Model file for the job. Use its own axes, mm. A direction names the side the tool comes from. Give positions to 0.01 mm unless a question says otherwise; leave off trailing zeros. Order: outer loops, then holes, each group sorted by start corner. A loop starts at its lowest first (then second) coordinate and runs counter-clockwise, first axis right, second up. Notation, with made-up numbers: M 3.5,-20 L 36.5,-20 A16 cw 36.5,-6 Z; hole C 46.25,80 d6. An arc over 180 degrees is marked long. Return JSON: item names as keys, results as strings. Group by question number.
1. Wall check: probe 1 along Z at (x, y) = (5.75, 2); probe 2 along X at (y, z) = (-4.4, 14.5); probe 3 along Z at (x, y) = (-10, 2.5). Give the ranges that are in metal, low to high. Write a range as [from, to].
2. Two-plate mould, pull along Y, no slides. Class faces 5 (the face through (7.5, -2.02, 15.97)), 6 (the face through (0, -6.5, 14)), 7 (the face through (0, 0, 2)), 8 (the face through (11, -0.5, 16)): released by +Y, released by -Y, zero draft, split by the parting line, or undercut.
3. Slice it at A-A on z = 12.5. List the corners of the cut face in (x, y), then the cut area to 3 significant figures.
4. 3-axis set-ups, long thin cutter, end or side, ignore diameter. For faces 1 (the face through (-1, -3, 7)), 2 (the face through (-10.97, -5.02, 13.23)), 3 (the face through (-7.477, -2.021, 15.93)), 4 (the face through (11, -2, 17.4)): which of +Z, -Z, +X, -X, +Y, -Y reach the whole face in a straight line?
5. Pin check, flat tips, straight feed: pin 1 (3 mm diameter, centred on x = 1.5, z = 12.5, fed in from +Y); pin 2 (0.9 mm diameter, centred on x = 12, y = -1.5, fed in from -Z); pin 3 (2.5 mm diameter, centred on x = -9.5, y = -2, fed in from +Z). Stop position of each tip, or through.
6. Slice it at B-B on z = 24.5. Give the number of separate pieces and of enclosed holes in the cut face, then the cut area to 3 significant figures.
from build123d import *

# Parameters (mm, degrees)
ESBO_O1_W                  = 26
ESBO_O1_H                  = 13
RESSALTO_EXTRUS_O1_DEPTH   = 29
CORTE_EXTRUS_O1_DEPTH      = 33.438403167
CORTE_EXTRUS_O1_DEPTH_BACK = 33.438403167
ESBO_O2_R                  = 5.5
ESBO_O3_R                  = 7.5
CORTE_EXTRUS_O2_DEPTH      = 25
CORTE_EXTRUS_O3_DEPTH      = 35.336569427
CORTE_EXTRUS_O3_DEPTH_BACK = 35.336569427
ESBO_O4_R                  = 1.6
CORTE_EXTRUS_O4_DEPTH      = 3
ESBO_O9_W                  = 8
ESBO_O9_H                  = 4
CORTE_EXTRUS_O5_DEPTH      = 3
FILETE1_R                  = 5


with BuildPart() as part:
    # Esboço1 → Ressalto-extrusão1 (new body)
    with BuildSketch(Plane.XY):
        Rectangle(ESBO_O1_W, ESBO_O1_H)
    extrude(amount=RESSALTO_EXTRUS_O1_DEPTH)

    # Esboço2 → Corte-extrusão1 (cut, two sides: drawn at the far end of the back side and taken through both)
    with BuildSketch(Plane.XY.offset(29).offset(-CORTE_EXTRUS_O1_DEPTH_BACK)):
        with Locations((0, 6.5)):
            Circle(ESBO_O2_R)
    extrude(amount=CORTE_EXTRUS_O1_DEPTH + CORTE_EXTRUS_O1_DEPTH_BACK, mode=Mode.SUBTRACT)

    # Esboço3 → Corte-extrusão2 (cut)
    with BuildSketch(Plane.XY.offset(27)):
        with Locations((0, 6.5)):
            Circle(ESBO_O3_R)
    extrude(amount=-CORTE_EXTRUS_O2_DEPTH, mode=Mode.SUBTRACT)

    # Esboço4 → Corte-extrusão3 (cut, two sides: drawn at the far end of the back side and taken through both)
    with BuildSketch(Plane(origin=(0, 6.5, 0), x_dir=(1, 0, 0), z_dir=(0, 1, 0)).offset(-CORTE_EXTRUS_O3_DEPTH_BACK)):
        with Locations(Location((-10, -14.5, 0), (0, 0, 270))):
            Circle(ESBO_O4_R)
        with Locations(Location((10, -14.5, 0), (0, 0, 270))):
            Circle(ESBO_O4_R)
    extrude(amount=CORTE_EXTRUS_O3_DEPTH + CORTE_EXTRUS_O3_DEPTH_BACK, mode=Mode.SUBTRACT)

    # Varredura de corte3: read off the stored shape, not the designer's step
    # Varredura de corte3: loft between two sections, ruled curve by curve
    varredura_de_corte3_from = [
        Edge.make_bspline([(-10.775531387, 11.14102753, 3), (-10.815047893, 10.387007675, 3), (-10.859579119, 9.537232339, 3), (-10.942482774, 7.955474229, 3), (-11.000003483, 7.230191203, 3), (-10.999993175, 5.06927711, 3), (-10.717078713, 3.385508213, 3), (-9.067866438, -0.006108266, 3), (-7.679635371, -1.685716419, 3), (-4.830903728, -3.44525385, 3), (-3.774716833, -3.895333549, 3), (-1.552511027, -4.449938605, 3), (-0.403453822, -4.550209028, 3), (2.969944564, -4.328615808, 3), (5.023571546, -3.476580102, 3), (8.13506471, -1.154366891, 3), (9.189674801, 0.267167465, 3), (10.533085234, 2.985384839, 3), (10.837160801, 4.285623822, 3), (11.004780041, 6.01871971, 3), (11.006990461, 6.575860832, 3), (10.96949773, 7.517101654, 3), (10.943022714, 7.945129378, 3), (10.873144208, 9.27841043, 3), (10.824758408, 10.201720017, 3), (10.775531387, 11.14102753, 3)], [0, 0, 0, 0, 0.056576928, 0.056576928, 0.113153857, 0.113153857, 0.224009625, 0.224009625, 0.334865393, 0.334865393, 0.390293276, 0.390293276, 0.44572116, 0.44572116, 0.556576928, 0.556576928, 0.667432696, 0.667432696, 0.778288464, 0.778288464, 0.833716348, 0.833716348, 0.889144232, 0.889144232, 1, 1, 1, 1], 3),
        Edge.make_bspline([(-8.778272317, 11.036355618, 3), (-8.818366558, 10.271311923, 3), (-8.86155068, 9.447238277, 3), (-8.945993073, 7.836124466, 3), (-9.000002401, 7.107268908, 3), (-8.999995296, 5.310128738, 3), (-8.764237068, 3.942975251, 3), (-7.423445328, 1.185624705, 3), (-6.27357029, -0.203437636, 3), (-3.957441466, -1.63400923, 3), (-3.084493861, -2.006248941, 3), (-1.274147115, -2.45806464, 3), (-0.32387933, -2.540671478, 3), (2.417516141, -2.360593842, 3), (4.119219834, -1.655921663, 3), (6.646937102, 0.230601396, 3), (7.51801706, 1.398774697, 3), (8.618786605, 3.626040825, 3), (8.867342653, 4.694186327, 3), (9.003623581, 6.103250891, 3), (9.006690622, 6.5435831, 3), (8.972969022, 7.390126226, 3), (8.946060492, 7.834793966, 3), (8.875291444, 9.185065517, 3), (8.82794518, 10.088540932, 3), (8.778272317, 11.036355618, 3)], [0, 0, 0, 0, 0.056576928, 0.056576928, 0.113153857, 0.113153857, 0.224009625, 0.224009625, 0.334865393, 0.334865393, 0.390293276, 0.390293276, 0.44572116, 0.44572116, 0.556576928, 0.556576928, 0.667432696, 0.667432696, 0.778288464, 0.778288464, 0.833716348, 0.833716348, 0.889144232, 0.889144232, 1, 1, 1, 1], 3),
        Edge.make_line((-8.778272317, 11.036355618, 3), (-10.775531387, 11.14102753, 3)),
        Edge.make_line((8.778272317, 11.036355618, 3), (10.775531387, 11.14102753, 3)),
    ]
    varredura_de_corte3_to = [
        Edge.make_bspline([(-10.775531387, 11.14102753, 7), (-10.815047893, 10.387007675, 7), (-10.859579119, 9.537232339, 7), (-10.942482774, 7.955474229, 7), (-11.000003483, 7.230191203, 7), (-10.999993175, 5.06927711, 7), (-10.717078713, 3.385508213, 7), (-9.067866438, -0.006108266, 7), (-7.679635371, -1.685716419, 7), (-4.830903728, -3.44525385, 7), (-3.774716833, -3.895333549, 7), (-1.552511027, -4.449938605, 7), (-0.403453822, -4.550209028, 7), (2.969944564, -4.328615808, 7), (5.023571546, -3.476580102, 7), (8.13506471, -1.154366891, 7), (9.189674801, 0.267167465, 7), (10.533085234, 2.985384839, 7), (10.837160801, 4.285623822, 7), (11.004780041, 6.01871971, 7), (11.006990461, 6.575860832, 7), (10.96949773, 7.517101654, 7), (10.943022714, 7.945129378, 7), (10.873144208, 9.27841043, 7), (10.824758408, 10.201720017, 7), (10.775531387, 11.14102753, 7)], [0, 0, 0, 0, 0.056576928, 0.056576928, 0.113153857, 0.113153857, 0.224009625, 0.224009625, 0.334865393, 0.334865393, 0.390293276, 0.390293276, 0.44572116, 0.44572116, 0.556576928, 0.556576928, 0.667432696, 0.667432696, 0.778288464, 0.778288464, 0.833716348, 0.833716348, 0.889144232, 0.889144232, 1, 1, 1, 1], 3),
        Edge.make_bspline([(-8.778272317, 11.036355618, 7), (-8.818366558, 10.271311923, 7), (-8.86155068, 9.447238277, 7), (-8.945993073, 7.836124466, 7), (-9.000002401, 7.107268908, 7), (-8.999995296, 5.310128738, 7), (-8.764237068, 3.942975251, 7), (-7.423445328, 1.185624705, 7), (-6.27357029, -0.203437636, 7), (-3.957441466, -1.63400923, 7), (-3.084493861, -2.006248941, 7), (-1.274147115, -2.45806464, 7), (-0.32387933, -2.540671478, 7), (2.417516141, -2.360593842, 7), (4.119219834, -1.655921663, 7), (6.646937102, 0.230601396, 7), (7.51801706, 1.398774697, 7), (8.618786605, 3.626040825, 7), (8.867342653, 4.694186327, 7), (9.003623581, 6.103250891, 7), (9.006690622, 6.5435831, 7), (8.972969022, 7.390126226, 7), (8.946060492, 7.834793966, 7), (8.875291444, 9.185065517, 7), (8.82794518, 10.088540932, 7), (8.778272317, 11.036355618, 7)], [0, 0, 0, 0, 0.056576928, 0.056576928, 0.113153857, 0.113153857, 0.224009625, 0.224009625, 0.334865393, 0.334865393, 0.390293276, 0.390293276, 0.44572116, 0.44572116, 0.556576928, 0.556576928, 0.667432696, 0.667432696, 0.778288464, 0.778288464, 0.833716348, 0.833716348, 0.889144232, 0.889144232, 1, 1, 1, 1], 3),
        Edge.make_line((-8.778272317, 11.036355618, 7), (-10.775531387, 11.14102753, 7)),
        Edge.make_line((8.778272317, 11.036355618, 7), (10.775531387, 11.14102753, 7)),
    ]
    varredura_de_corte3 = Solid(Shell([*[Face.make_surface_from_curves(varredura_de_corte3_from[k], varredura_de_corte3_to[k]) for k in range(4)], Face(Wire(varredura_de_corte3_from)), Face(Wire(varredura_de_corte3_to))]))
    add(varredura_de_corte3, mode=Mode.SUBTRACT)

    # Varredura de corte3 2: loft between two sections, ruled curve by curve
    varredura_de_corte3_2_from = [
        Edge.make_bspline([(-10.775531387, 11.14102753, 22), (-10.815050253, 10.386962648, 22), (-10.859635544, 9.536156226, 22), (-10.942604964, 7.953142141, 22), (-11.000003387, 7.227604876, 22), (-10.999993448, 5.09243912, 22), (-10.726075216, 3.44374676, 22), (-9.146415207, 0.117814577, 22), (-7.826638231, -1.531050563, 22), (-4.171497206, -3.909251659, 22), (-1.912358031, -4.556779213, 22), (2.517456834, -4.434897746, 22), (4.570919991, -3.689422793, 22), (7.764052722, -1.527285148, 22), (8.887440792, -0.158899703, 22), (10.364225069, 2.511206921, 22), (10.732123337, 3.816518914, 22), (10.975605623, 5.5614094, 22), (11.004902153, 6.119453759, 22), (10.993656399, 7.13678057, 22), (10.963259766, 7.559009248, 22), (10.895302463, 8.855554069, 22), (10.847393897, 9.769809145, 22), (10.799382035, 10.685930053, 22)], [0, 0, 0, 0, 0.057220999, 0.057220999, 0.114441998, 0.114441998, 0.225136749, 0.225136749, 0.335831499, 0.335831499, 0.446526249, 0.446526249, 0.557220999, 0.557220999, 0.667915749, 0.667915749, 0.7786105, 0.7786105, 0.833957875, 0.833957875, 0.88930525, 0.88930525, 1, 1, 1, 1], 3),
        Edge.make_bspline([(-8.778272317, 11.036355618, 22), (-8.818364203, 10.271356871, 22), (-8.861613386, 9.446042366, 22), (-8.946108983, 7.833912176, 22), (-9.000002332, 7.104831646, 22), (-8.999995488, 5.329945493, 22), (-8.772011309, 3.991285732, 22), (-7.487299037, 1.286355363, 22), (-6.385007619, -0.082964565, 22), (-3.431648648, -2.004555434, 22), (-1.541287594, -2.5458131, 22), (2.036368433, -2.447377138, 22), (3.749427608, -1.830311698, 22), (6.342822793, -0.074267526, 22), (7.271131746, 1.051066146, 22), (8.480231231, 3.237185214, 22), (8.780527991, 4.302274211, 22), (8.980191062, 5.733137414, 22), (9.004131059, 6.178194136, 22), (8.994672137, 7.033801275, 22), (8.966591972, 7.443057915, 22), (8.896860843, 8.773440999, 22), (8.851022767, 9.64819435, 22), (8.802122965, 10.58125814, 22)], [0, 0, 0, 0, 0.057220999, 0.057220999, 0.114441998, 0.114441998, 0.225136749, 0.225136749, 0.335831499, 0.335831499, 0.446526249, 0.446526249, 0.557220999, 0.557220999, 0.667915749, 0.667915749, 0.7786105, 0.7786105, 0.833957875, 0.833957875, 0.88930525, 0.88930525, 1, 1, 1, 1], 3),
        Edge.make_line((-8.778272317, 11.036355618, 22), (-10.775531387, 11.14102753, 22)),
        Edge.make_line((8.802122965, 10.58125814, 22), (10.799382035, 10.685930053, 22)),
    ]
    varredura_de_corte3_2_to = [
        Edge.make_bspline([(-10.775531387, 11.14102753, 26), (-10.815050253, 10.386962648, 26), (-10.859635544, 9.536156226, 26), (-10.942604964, 7.953142141, 26), (-11.000003387, 7.227604876, 26), (-10.999993448, 5.09243912, 26), (-10.726075216, 3.44374676, 26), (-9.146415207, 0.117814577, 26), (-7.826638231, -1.531050563, 26), (-4.171497206, -3.909251659, 26), (-1.912358031, -4.556779213, 26), (2.517456834, -4.434897746, 26), (4.570919991, -3.689422793, 26), (7.764052722, -1.527285148, 26), (8.887440792, -0.158899703, 26), (10.364225069, 2.511206921, 26), (10.732123337, 3.816518914, 26), (10.975605623, 5.5614094, 26), (11.004902153, 6.119453759, 26), (10.993656399, 7.13678057, 26), (10.963259766, 7.559009248, 26), (10.895302463, 8.855554069, 26), (10.847393897, 9.769809145, 26), (10.799382035, 10.685930053, 26)], [0, 0, 0, 0, 0.057220999, 0.057220999, 0.114441998, 0.114441998, 0.225136749, 0.225136749, 0.335831499, 0.335831499, 0.446526249, 0.446526249, 0.557220999, 0.557220999, 0.667915749, 0.667915749, 0.7786105, 0.7786105, 0.833957875, 0.833957875, 0.88930525, 0.88930525, 1, 1, 1, 1], 3),
        Edge.make_bspline([(-8.778272317, 11.036355618, 26), (-8.818364203, 10.271356871, 26), (-8.861613386, 9.446042366, 26), (-8.946108983, 7.833912176, 26), (-9.000002332, 7.104831646, 26), (-8.999995488, 5.329945493, 26), (-8.772011309, 3.991285732, 26), (-7.487299037, 1.286355363, 26), (-6.385007619, -0.082964565, 26), (-3.431648648, -2.004555434, 26), (-1.541287594, -2.5458131, 26), (2.036368433, -2.447377138, 26), (3.749427608, -1.830311698, 26), (6.342822793, -0.074267526, 26), (7.271131746, 1.051066146, 26), (8.480231231, 3.237185214, 26), (8.780527991, 4.302274211, 26), (8.980191062, 5.733137414, 26), (9.004131059, 6.178194136, 26), (8.994672137, 7.033801275, 26), (8.966591972, 7.443057915, 26), (8.896860843, 8.773440999, 26), (8.851022767, 9.64819435, 26), (8.802122965, 10.58125814, 26)], [0, 0, 0, 0, 0.057220999, 0.057220999, 0.114441998, 0.114441998, 0.225136749, 0.225136749, 0.335831499, 0.335831499, 0.446526249, 0.446526249, 0.557220999, 0.557220999, 0.667915749, 0.667915749, 0.7786105, 0.7786105, 0.833957875, 0.833957875, 0.88930525, 0.88930525, 1, 1, 1, 1], 3),
        Edge.make_line((-8.778272317, 11.036355618, 26), (-10.775531387, 11.14102753, 26)),
        Edge.make_line((8.802122965, 10.58125814, 26), (10.799382035, 10.685930053, 26)),
    ]
    varredura_de_corte3_2 = Solid(Shell([*[Face.make_surface_from_curves(varredura_de_corte3_2_from[k], varredura_de_corte3_2_to[k]) for k in range(4)], Face(Wire(varredura_de_corte3_2_from)), Face(Wire(varredura_de_corte3_2_to))]))
    add(varredura_de_corte3_2, mode=Mode.SUBTRACT)

    # Esboço8 → Corte-extrusão4 (cut)
    with BuildSketch(Plane(origin=(0, -3.5, 0), x_dir=(-1, 0, 0), z_dir=(0, -1, 0))):
        Polygon((-11.674315781, -11.6), (-15.702583778, -11.6), (-15.702583778, -17.4), (-11.674315781, -17.4), (-8.325684219, -17.4), (-6.651368439, -14.5), (-8.325684219, -11.6), align=None)
        Polygon((11.674315781, -11.6), (8.325684219, -11.6), (6.651368439, -14.5), (8.325684219, -17.4), (11.674315781, -17.4), (15.292356459, -17.4), (15.292356459, -11.6), align=None)
    extrude(amount=-CORTE_EXTRUS_O4_DEPTH, mode=Mode.SUBTRACT)

    # Esboço9 → Corte-extrusão5 (cut)
    with BuildSketch(Plane.XZ.offset(6.5)):
        with Locations((0, 24)):
            Rectangle(ESBO_O9_W, ESBO_O9_H)
        with Locations((0, 5)):
            Rectangle(ESBO_O9_W, ESBO_O9_H)
    extrude(amount=-CORTE_EXTRUS_O5_DEPTH, mode=Mode.SUBTRACT)

    # Filete1
    filete1_edges = [part.edges().sort_by_distance(p)[0] for p in [
        (-13, 0, 29),
        (13, 0, 29),
        (-13, 0, 0),
        (13, 0, 0),
    ]]
    fillet(filete1_edges, radius=FILETE1_R)


solid = part.part
Result:
{
 "1": {"probe 1": "z = [0, 2], [27, 29]", "probe 2": "x = [-13, -11.6], [-8.4, 8.4], [11.6, 13]", "probe 3": "z = [0.42, 3], [7, 12.9], [16.1, 22], [26, 28.58]"},
 "2": {"face 5": "undercut", "face 6": "released by -Y", "face 7": "zero draft", "face 8": "undercut"},
 "3": {"outline": "M -13,-6.5 L 13,-6.5 L 13,-3.5 L 7.81,-3.5 L 7.81,-0.5 L 13,-0.5 L 13,6.5 L 7.5,6.5 A7.5 cw -7.5,6.5 L -13,6.5 L -13,-0.5 L -7.81,-0.5 L -7.81,-3.5 L -13,-3.5 Z", "area": "218 mm2"},
 "4": {"face 1": "none", "face 2": "+Y, -Y", "face 3": "-X", "face 4": "+X"},
 "5": {"pin 1": "stops at y = -0.37", "pin 2": "stops at z = 1.48", "pin 3": "stops at z = 28.99"},
 "6": {"separate pieces": "3", "enclosed holes": "0", "area": "168 mm2"}
}
